Verification items for this drawing (mm, ordinates from the low corner). Round coordinates to 2 decimals unless told otherwise and drop trailing zeros. Loops run counter-clockwise (first coordinate to the right, second up) from the corner with the lowest first, then second, coordinate; pieces in that order, holes last. Notation, with made-up numbers: M 80.5,20.5 L 123.5,20.5 A18 ccw 123.5,50.5 Z; hole C 43,-21 d10. An arc over 180 degrees is marked long. Write item = value, one per line. Start each with the question number.
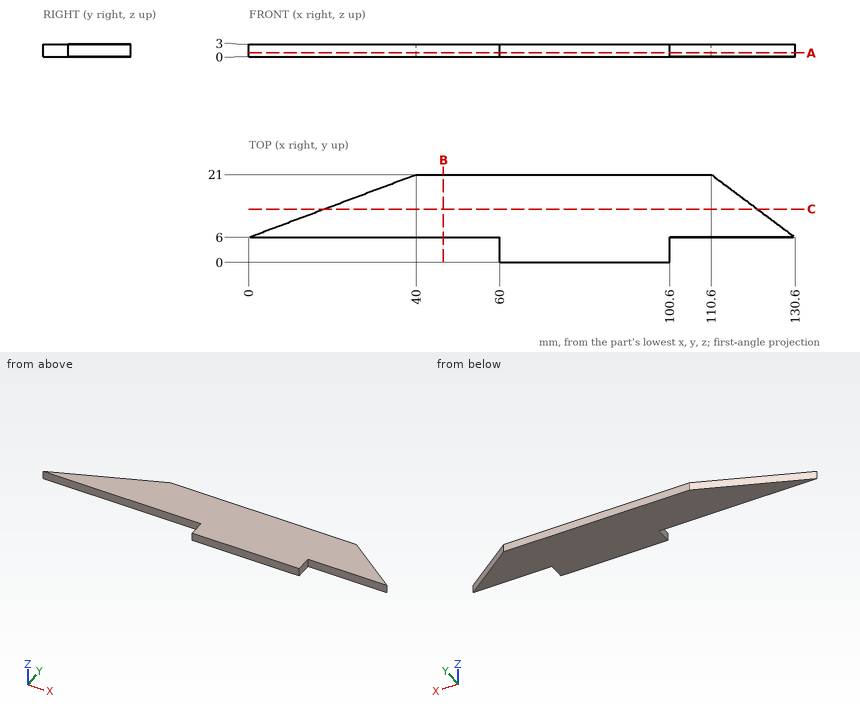
1. Gauge pin test, flat ends, axial feed: P1, Ø1.5, axis at y = 4.5, z = 1, coming from the -X side; P2, Ø1.5, axis at x = 118.5, z = 1, coming from the -Y side. Record the tip position at first contact, or that the pin passes through.
2. Section check B-B, the plane x = 46.5. Enter the section's corners in (y, z).
3. Thickness scan on line 1 (Y direction, x = 50, z = 2.75); line 2 (X direction, y = 5, z = 2.4); line 3 (Y direction, x = 39, z = 0.5) (3 decimals). Record the ranges inside material, lowest first.
4. Section check A-A, the plane z = 0.9. Enter the section's corners in (x, y), and give its area (3 significant figures).
5. Section check C-C, the plane y = 12.75. Enter the section's corners in (x, z), and give its area (3 significant figures).
Computed values:
q1.P1 = 60
q1.P2 = 6
q2.outline = M 6,0 L 21,0 L 21,3 L 6,3 Z
q3.line_1 = 6 to 21
q3.line_2 = 60 to 100.6
q3.line_3 = 6 to 20.625
q4.outline = M 0,6 L 60,6 L 60,0 L 100.6,0 L 100.6,6 L 130.6,6 L 110.6,21 L 40,21 Z
q4.area = 1,750 mm2
q5.outline = M 18,0 L 121.6,0 L 121.6,3 L 18,3 Z
q5.area = 311 mm2
